Geometry: final body of the model. Coordinates: model frame, mm. A direction names the side the tool comes from. Round coordinates to 2 decimals unless told otherwise and drop trailing zeros. Loops run counter-clockwise (first coordinate to the right, second up) from the corner with the lowest first, then second, coordinate; pieces in that order, holes last. Notation, with made-up numbers: (-17.75, 52.5) - (-7.75, 52.5) arc R19 ccw to (-7.75, 64.5) - close; hole circle Ø9 at (-19.5, -10.75). An arc over 180 degrees is marked (long way). Answer as a JSON object with one key per item and string values. Group by question number.
Item 1: Line query: line 1 (X direction, y = 0.25, z = 4.25); line 2 (Z direction, x = 5.5, y = 0); line 3 (Y direction, x = 6.75, z = -4). Output: solid intervals per line, ascending.
Item 2: Section A-A (y = 0). Return the cut outline in (x, z) (3 decimals).
Item 3: First-contact query: pin 1 (4 mm diameter, centred on x = 5.5, y = 4, fed in from -Z); pin 2 (1.5 mm diameter, centred on x = 2.5, y = 1, fed in from +Z); pin 3 (6 mm diameter, centred on y = 0, z = 0, fed in from -X); pin 4 (2 mm diameter, centred on x = 2, z = -3.5, fed in from +Y). Flat tips, straight axial feed; report the tip coordinate or a pass-through.
Item 4: Draft query along X for faces 3 (the face through (0, -3.2, -2.1)), 4 (the face through (0.254, -0.797, -3.588)), 5 (the face through (0.5, -3.2, -2.1)). Return one class per face: released by +X, released by -X, zero draft, split by the parting line, or undercut.
Item 5: Section C-C (x = 2). Return the cut outline in (y, z).
Item 6: Reachability of faces 1 (the face through (9, -3.2, -2.1)), 2 (the face through (8.5, -3.2, -2.1)) from +Z, -Z, +X, -X, +Y, -Y: full face, straight path, thin tool, end or side. Return the list, or none.
Autodesk Inventor part; units mm, degrees
ref_plane "IP_1_XY" through (0, 0, 0) normal (1, 0, 0) x (0, 0, -1)
ref_plane "IP_1_YZ" through (0, 0, 0) normal (0, 0, -1) x (0, 1, 0)
ref_plane "IP_1_ZX" through (0, 0, 0) normal (0, 1, 0) x (1, 0, 0)
sketch "Sketch_1" plane through (0, 0, 0) normal (0, 0, 1) x (1, 0, 0)
  line L0 (9, 0) -> (0, 0)
  line L1 (0, 3.675) -> (0.5, 3.675)
  line L2 (0.5, 3.675) -> (0.5, 4.7)
  arc A0 (0.8, 5) -> (0.5, 4.7) centre (0.8, 4.7) ccw
  line L3 (0.8, 5) -> (8.2, 5)
  arc A1 (8.5, 4.7) -> (8.2, 5) centre (8.2, 4.7) ccw
  line L4 (8.5, 4.7) -> (8.5, 3.675)
  line L5 (8.5, 3.675) -> (9, 3.675)
  line L6 (9, 3.675) -> (9, 4.7)
  arc A2 (9, 4.7) -> (8.2, 5.5) centre (8.2, 4.7) ccw
  line L7 (8.2, 5.5) -> (0.8, 5.5)
  arc A3 (0.8, 5.5) -> (0, 4.7) centre (0.8, 4.7) ccw
  line L8 (0, 4.7) -> (0, 3.675)
revolve "Revolution1" add sketch "Sketch_1" angle 360 about axis through (9, 0, 0) along (1, 0, 0)
ref_plane "IP_1_XY" through (0, 0, 0) normal (1, 0, 0) x (0, 0, -1)
ref_plane "IP_1_YZ" through (0, 0, 0) normal (0, 0, -1) x (0, 1, 0)
ref_plane "IP_1_ZX" through (0, 0, 0) normal (0, 1, 0) x (1, 0, 0)
ref_plane "IP_5_XY" through (4.5, 0, 0) normal (1, 0, 0) x (0, 0, -1)
ref_plane "IP_5_YZ" through (4.5, 0, 0) normal (0, 0, -1) x (0, 1, 0)
ref_plane "IP_5_ZX" through (4.5, 0, 0) normal (0, 1, 0) x (1, 0, 0)
ref_plane "IP_6_XY" through (6.35, 0, 0) normal (1, 0, 0) x (0, 0, -1)
ref_plane "IP_6_YZ" through (6.35, 0, 0) normal (0, 0, -1) x (0, 1, 0)
ref_plane "IP_6_ZX" through (6.35, 0, 0) normal (0, 1, 0) x (1, 0, 0)
properties part number "HK0709FMSH" material "Steel"
Values:
{
 "1": {"line 1": "x = 0 to 0.5, 8.5 to 9", "line 2": "z = -5.5 to -5, 5 to 5.5", "line 3": "y = -3.77 to -3, 3 to 3.77"},
 "2": {"outline": "(0, -4.7) arc R0.8 ccw to (0.8, -5.5) - (8.2, -5.5) arc R0.8 ccw to (9, -4.7) - (9, -3.675) - (8.5, -3.675) - (8.5, -4.7) arc R0.3 cw to (8.2, -5) - (0.8, -5) arc R0.3 cw to (0.5, -4.7) - (0.5, -3.675) - (0, -3.675) - close; (0, 3.675) - (0.5, 3.675) - (0.5, 4.7) arc R0.3 cw to (0.8, 5) - (8.2, 5) arc R0.3 cw to (8.5, 4.7) - (8.5, 3.675) - (9, 3.675) - (9, 4.7) arc R0.8 ccw to (8.2, 5.5) - (0.8, 5.5) arc R0.8 ccw to (0, 4.7) - close"},
 "3": {"pin 1": "stops at z = -5.12", "pin 2": "stops at z = 5.49", "pin 3": "passes through", "pin 4": "stops at y = 4.9"},
 "4": {"face 3": "released by -X", "face 4": "zero draft", "face 5": "undercut"},
 "5": {"outline": "circle Ø11 at (0, 0); hole circle Ø10 at (0, 0)"},
 "6": {"face 1": "+Z, -Z, +X, +Y, -Y", "face 2": "none"}
}
